Geometry check sheet. Reference: the model listing, model coordinates, mm. Face numbers are marked on the shaded views. A direction names the side the tool comes from. Round coordinates to 2 decimals unless told otherwise and drop trailing zeros. Order: outer loops, then holes, each group sorted by start corner. A loop starts at its lowest first (then second) coordinate and runs counter-clockwise, first axis right, second up. Notation, with made-up numbers: (-19, 69.25) - (8, 69.25) arc R23 ccw to (8, 97.25) - close; hole circle Ø3 at (-24.5, 30.5). An arc over 180 degrees is marked (long way). Write each question's results on one line, items separated by ' | '.
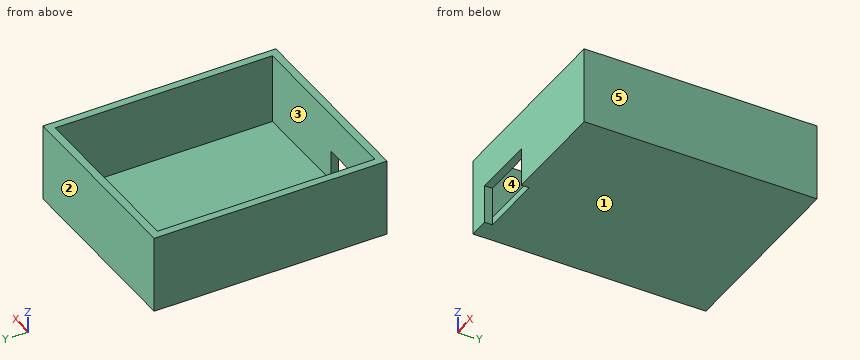
```python
from build123d import *

# Parameters (mm, degrees)
F0_W     = 63.5
F0_H     = 25.4
F1_DEPTH = 38.1
F2_T     = -2.54
F3_W     = 21.006488
F3_H     = 12.7
F4_DEPTH = 2.54


with BuildPart() as f1:
    # F0 (on Front) → F1 (new body, symmetric)
    with BuildSketch(Plane.XZ):
        with Locations((-20.382458, 12.7)):
            Rectangle(F0_W, F0_H)
    extrude(amount=F1_DEPTH, both=True)

    # F2
    f2_openings = [f1.faces().sort_by_distance(p)[0] for p in [
        (-20.382458, 0, 25.4),
    ]]
    offset(amount=F2_T, openings=f2_openings)

    # F3 (on face) → F4 (cut)
    with BuildSketch(Plane.XZ.offset(38.1)):
        with Locations((-35.010811, 6.35)):
            Rectangle(F3_W, F3_H)
    extrude(amount=-F4_DEPTH, mode=Mode.SUBTRACT)


solid = f1.part
```
(1) Depth check by flat-ended pin: pin 1 Ø3 at (x, y) = (-39.5, -23) entering from +Z; pin 2 Ø2 at (x, z) = (-39.5, 1.5) entering from -Y; pin 3 Ø0.8 at (x, y) = (-36.5, -36.5) entering from -Z. Enter the tip coordinate at first touch or a pass-through.
Answers follow:
pin 1: z = 2.54 | pin 2: y = -35.56 | pin 3: z = 12.7
(2) Draft check along Y on the marked faces 1, 2 and 3. Enter one of: released by +Y, released by -Y, zero draft, split by the parting line, or undercut.
Answers follow:
face 1: zero draft | face 2: released by +Y | face 3: undercut
(3) Section check B-B (z = 4.75). Record the cut outline in (x, y).
Answers follow:
outline: (-52.13, -38.1) - (-45.51, -38.1) - (-45.51, -35.56) - (-49.59, -35.56) - (-49.59, 35.56) - (8.83, 35.56) - (8.83, -35.56) - (-24.51, -35.56) - (-24.51, -38.1) - (11.37, -38.1) - (11.37, 38.1) - (-52.13, 38.1) - close
(4) Section check D-D (x = -9.5). Record the cut outline in (y, z), then the cut area to 3 significant figures.
Answers follow:
outline: (-38.1, 0) - (38.1, 0) - (38.1, 25.4) - (35.56, 25.4) - (35.56, 2.54) - (-35.56, 2.54) - (-35.56, 25.4) - (-38.1, 25.4) - close | area: 310 mm²
(5) Section check C-C (y = -8.5). Record the cut outline in (x, z), then the cut area to 3 significant figures.
Answers follow:
outline: (-52.13, 0) - (11.37, 0) - (11.37, 25.4) - (8.83, 25.4) - (8.83, 2.54) - (-49.59, 2.54) - (-49.59, 25.4) - (-52.13, 25.4) - close | area: 277 mm²
(6) Access from +Z, -Z, +X, -X, +Y, -Y to the whole of each face (thin tool, end or side, straight path). Record for the marked faces 4 and 5.
Answers follow:
face 4: +Z | face 5: +Z, -Z, +X, +Y, -Y
(7) Section check A-A (x = -28). Record the cut outline in (y, z), then the cut area to 3 significant figures.
Answers follow:
outline: (-38.1, 12.7) - (-35.56, 12.7) - (-35.56, 25.4) - (-38.1, 25.4) - close; (-35.56, 0) - (38.1, 0) - (38.1, 25.4) - (35.56, 25.4) - (35.56, 2.54) - (-35.56, 2.54) - close | area: 277 mm²
(8) Material ranges on line 1 (Y direction, x = -20.5, z = 7.5); line 2 (X direction, y = -6.5, z = 14.75); line 3 (Z direction, x = -19, y = 15.5), recorded low to high.
Answers follow:
line 1: -38.1 to -35.56, 35.56 to 38.1 | line 2: -52.13 to -49.59, 8.83 to 11.37 | line 3: 0 to 2.54
